Design review of the part built by this model. Coordinates are the model's own, in mm. A direction names the side the tool comes from. Coordinates: 2 decimals unless noted, no trailing zeros. Order: outer loops, then holes, each group sorted by start corner. A loop starts at its lowest first (then second) coordinate and runs counter-clockwise, first axis right, second up. Notation, with made-up numbers: (0, 2) -> (49, 2) arc R18 ccw to (49, 11) -> close; hole circle Ø10 at (20.5, 29). An arc over 180 degrees is marked (long way). Write item = value, one per line.
```python
from build123d import *

# Parameters (mm, degrees)
F0_R     = 7.55
F1_DEPTH = 10
F0_W     = 10
F0_H     = 10
F0_R_2   = 2.5
F2_DEPTH = 5
F3_DEPTH = 15
F4_DEPTH = 10


with BuildPart() as f1:
    # F0 (on Top) → F1 (new body)
    with BuildSketch(Plane.XY):
        Polygon((10, -10), (10, 10), (-10, 10), (-10, -10), (0, -10), align=None)
        Circle(F0_R, mode=Mode.SUBTRACT)
    extrude(amount=F1_DEPTH)

    # F0 (on Top) → F2 (join)
    with BuildSketch(Plane.XY):
        with Locations((-5, -15)):
            Rectangle(F0_W, F0_H)
        with Locations((-5, -15)):
            Circle(F0_R_2, mode=Mode.SUBTRACT)
        Polygon((10, -30), (10, -20), (0, -20), (-10, -20), (-10, -30), (-5, -30), (-5, -25), (5, -25), (5, -30), align=None)
        with Locations((-5, -15)):
            Circle(F0_R_2)
    extrude(amount=F2_DEPTH)

    # F0 (on Top) → F3 (join)
    with BuildSketch(Plane.XY):
        with Locations((5, -15)):
            Rectangle(F0_W, F0_H)
        with Locations((5, -15)):
            Circle(F0_R_2, mode=Mode.SUBTRACT)
    extrude(amount=F3_DEPTH)

    # F0 (on Top) → F4 (join)
    with BuildSketch(Plane.XY):
        with Locations((-5, -15)):
            Circle(F0_R_2)
    extrude(amount=F4_DEPTH)


solid = f1.part
```
(1) For L1, parallel to Y at x = 5, z = 10.25; L2, parallel to X at y = -11, z = 6; L3, parallel to Y at x = -6.75, z = 8.75, list the stretches that pass through material, from the lowest coordinate up.
Report:
L1 = -20 to -17.5, -12.5 to -10
L2 = 0 to 10
L3 = -16.79 to -13.21, -10 to -3.38, 3.38 to 10
(2) For faces 5 (the flat face through (-5, -15, 10)), 6 (the flat face through (0, -15, 10)), 7 (the flat face through (5, -10, 12)), 8 (the cylindrical face through (-2.69, -15.96, 7.46)), list the 3-axis set-ups (+Z, -Z, +X, -X, +Y, -Y) from which the entire face can be reached by the end or side of a thin tool; tool diameter is ignored.
Report:
face_5 = +Z, -X, +Y, -Y
face_6 = +Z, -Y
face_7 = +Z, +X, -X, +Y
face_8 = +Z
(3) The part is to be moulded in two halves that separate along X. For faces 1 (the flat face through (5, -27, 2)), 2 (the flat face through (10, -10, 6)), 3 (the flat face through (-5, -28, 2)), 4 (the flat face through (-8, -30, 2)), say which applies: released by +X, released by -X, zero draft, split by the parting line, or undercut.
Report:
face_1 = undercut
face_2 = released by +X
face_3 = undercut
face_4 = zero draft
(4) We need section C-C (x = -3). Write out the cut boundary in (y, z).
Report:
outline = (-25, 0) -> (-6.93, 0) -> (-6.93, 10) -> (-10, 10) -> (-10, 5) -> (-13.5, 5) -> (-13.5, 10) -> (-16.5, 10) -> (-16.5, 5) -> (-25, 5) -> close; (6.93, 0) -> (10, 0) -> (10, 10) -> (6.93, 10) -> close
(5) We need section A-A (z = 7.75). Write out the cut boundary in (x, y).
Report:
outline = (-10, -10) -> (0, -10) -> (0, -20) -> (10, -20) -> (10, 10) -> (-10, 10) -> close; circle Ø5 at (-5, -15); hole circle Ø15.1 at (0, 0); hole circle Ø5 at (5, -15)
(6) We need section D-D (z = 4.25). Write out the cut boundary in (x, y).
Report:
outline = (-10, -30) -> (-5, -30) -> (-5, -25) -> (5, -25) -> (5, -30) -> (10, -30) -> (10, 10) -> (-10, 10) -> close; hole circle Ø15.1 at (0, 0); hole circle Ø5 at (5, -15)
(7) Insertion check: pin 1 (2.5 mm diameter, centred on x = 3, z = 13, fed in from +Y); pin 2 (4 mm diameter, centred on x = -1, z = 2, fed in from -Y); pin 3 (10 mm diameter, centred on x = 3, y = 0.5, fed in from +Z); pin 4 (8 mm diameter, centred on x = -6.5, y = -14.5, fed in from -Z). Each pin has a flat end and moves straight along its axis. Give the tip position at first contact, or say it passes through.
Report:
pin_1 = -10
pin_2 = -25
pin_3 = 10
pin_4 = 0
(8) We need section B-B (y = 0). Write out the cut boundary in (x, z).
Report:
outline = (-10, 0) -> (-7.55, 0) -> (-7.55, 10) -> (-10, 10) -> close; (7.55, 0) -> (10, 0) -> (10, 10) -> (7.55, 10) -> close
